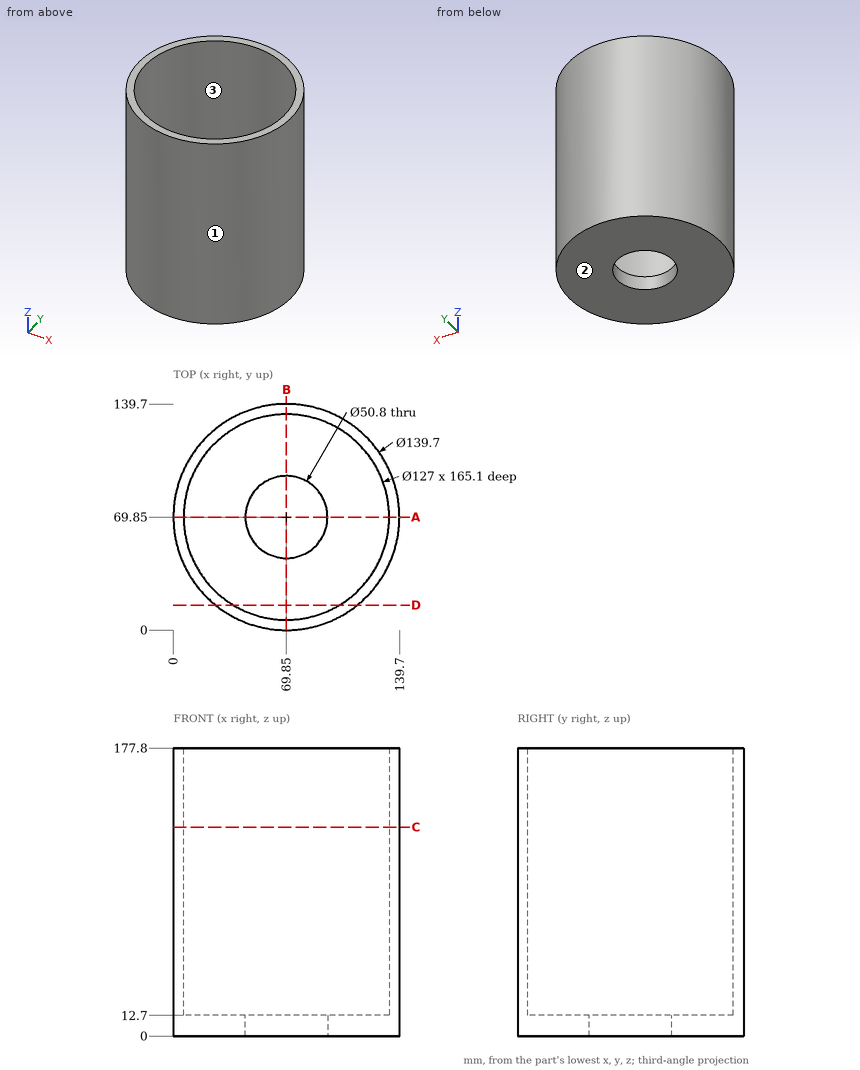
The drawing under review shows one solid part. Ordinate dimensions are in mm from its lowest x, y, z. Give positions to 0.01 mm unless a question says otherwise; leave off trailing zeros. Write each loop counter-clockwise with the first axis right and the second up, starting at its lowest first coordinate (ties: lowest second). Pieces come first, ordered by that corner, then holes.
1. Add section A-A, the plane y = 69.85. Write out the cut boundary in (x, z), plus the area to 3 significant figures.
2. Wall thickness on L1, parallel to X at y = 69, z = 9; L2, parallel to Y at x = 69, z = 145; L3, parallel to Y at x = 69.85, z = 3.5: over which ranges is each line inside the solid? List them lowest first.
3. Add section D-D, the plane y = 15.5. Write out the cut boundary in (x, z), plus the area to 3 significant figures.
4. Add section C-C, the plane z = 129. Write out the cut boundary in (x, y).
5. For P1, Ø8, axis at y = 54.5, z = 132.5, coming from the -X side; P2, Ø3, axis at x = 18.5, z = 113.5, coming from the -Y side; P3, Ø10, axis at x = 92, z = 100.5, coming from the +Y side, all flat-tipped, find the tip position at first contact; note any pin that passes through.
6. Draft analysis for pull direction Y (two halves, no side actions). For the marked faces 1, 2 and 3, state which applies: +Y half, -Y half, draft (parallel to the pull), parting line (faces both ways), or undercut.
Worked answers:
1. outline: (0, 0) - (44.45, 0) - (44.45, 12.7) - (6.35, 12.7) - (6.35, 177.8) - (0, 177.8) - close; (95.25, 0) - (139.7, 0) - (139.7, 177.8) - (133.35, 177.8) - (133.35, 12.7) - (95.25, 12.7) - close
1. area: 3,230 mm2
2. L1: x = 0.01 to 44.46, 95.24 to 139.69
2. L2: y = 0.01 to 6.36, 133.34 to 139.69
2. L3: y = 0 to 44.45, 95.25 to 139.7
3. outline: (25.97, 0) - (113.73, 0) - (113.73, 177.8) - (102.69, 177.8) - (102.69, 12.7) - (37.01, 12.7) - (37.01, 177.8) - (25.97, 177.8) - close
3. area: 4,760 mm2
4. outline: circle Ø139.7 at (69.85, 69.85); hole circle Ø127 at (69.85, 69.85)
5. P1: stops at x = 0.93
5. P2: stops at y = 20.92
5. P3: stops at y = 137.56
6. face 1: parting line
6. face 2: draft
6. face 3: undercut
